Design review of the part built by this model. Coordinates are the model's own, in mm. A direction names the side the tool comes from. Give positions to 0.01 mm unless a question says otherwise; leave off trailing zeros. Order: outer loops, then holes, each group sorted by start corner. A loop starts at its lowest first (then second) coordinate and runs counter-clockwise, first axis right, second up. Notation, with made-up numbers: M 46,44 L 70,44 A13 cw 70,48 Z; hole C 7.5,46.5 d6. An arc over 180 degrees is marked long. Answer as a JSON object with one key per item and string values.
from build123d import *

# Parameters (mm, degrees)
BOX_W           = 67
BOX_H           = 24.4
BOX_DEPTH       = 10.5
THICKNESS_T     = 1.2
SKETCH_W        = 8
SKETCH_H        = 4.3
POCKET_DEPTH    = 5
SKETCH001_W     = 15.5
SKETCH001_H     = 3.2
POCKET001_DEPTH = 5
SKETCH002_W     = 5
SKETCH002_H     = 1
PAD_DEPTH       = 0.5
SKETCH003_W     = 5
SKETCH003_H     = 1
PAD001_DEPTH    = 0.5
CHAMFER_SIZE    = 0.4
CHAMFER001_SIZE = 0.4
CHAMFER002_SIZE = 0.4
CHAMFER003_SIZE = 0.4


with BuildPart() as part:
    # Box → Box (new body)
    with BuildSketch(Plane.XY):
        with Locations((33.5, 12.2)):
            Rectangle(BOX_W, BOX_H)
    extrude(amount=BOX_DEPTH)

    # Thickness
    thickness_openings = [part.faces().sort_by_distance(p)[0] for p in [
        (33.5, 12.2, 10.5),
    ]]
    offset(amount=THICKNESS_T, openings=thickness_openings)

    # Sketch (on Face14 of Thickness) → Pocket (cut)
    with BuildSketch(Plane.XZ.offset(1.2)):
        with Locations((21.188957, 4.340102)):
            Rectangle(SKETCH_W, SKETCH_H)
    extrude(amount=-POCKET_DEPTH, mode=Mode.SUBTRACT)

    # Sketch001 (on Face17 of Pocket) → Pocket001 (cut)
    with BuildSketch(Plane.YZ.offset(68.2)):
        with Locations((15.481014, 3.816542)):
            Rectangle(SKETCH001_W, SKETCH001_H)
    extrude(amount=-POCKET001_DEPTH, mode=Mode.SUBTRACT)

    # Sketch002 (on Face2 of Pocket001) → Pad (join)
    with BuildSketch(Plane.XZ):
        with Locations((7.5565, 3.152776)):
            Rectangle(SKETCH002_W, SKETCH002_H)
        with Locations((62.523926, 3.21387)):
            Rectangle(SKETCH002_W, SKETCH002_H)
    extrude(amount=-PAD_DEPTH)

    # Sketch003 (on Face5 of Pad) → Pad001 (join)
    with BuildSketch(Plane(origin=(0, 24.4, 0), x_dir=(-1, 0, 0), z_dir=(0, 1, 0))):
        with Locations((-57.564125, 3.224103)):
            Rectangle(SKETCH003_W, SKETCH003_H)
        with Locations((-12.49075, 3.224103)):
            Rectangle(SKETCH003_W, SKETCH003_H)
    extrude(amount=-PAD001_DEPTH)

    # Chamfer
    chamfer_edges = [part.edges().sort_by_distance(p)[0] for p in [
        (12.49075, 23.9, 3.724103),
    ]]
    chamfer(chamfer_edges, length=CHAMFER_SIZE)

    # Chamfer001
    chamfer001_edges = [part.edges().sort_by_distance(p)[0] for p in [
        (57.564125, 23.9, 3.724103),
    ]]
    chamfer(chamfer001_edges, length=CHAMFER001_SIZE)

    # Chamfer002
    chamfer002_edges = [part.edges().sort_by_distance(p)[0] for p in [
        (62.523926, 0.5, 3.71387),
    ]]
    chamfer(chamfer002_edges, length=CHAMFER002_SIZE)

    # Chamfer003
    chamfer003_edges = [part.edges().sort_by_distance(p)[0] for p in [
        (7.5565, 0.5, 3.652776),
    ]]
    chamfer(chamfer003_edges, length=CHAMFER003_SIZE)


solid = part.part
(1) We need section A-A (z = 7.75). Write out the cut boundary in (x, y), plus the area to 3 significant figures.
Checked values:
{"outline": "M -1.2,0 A1.2 ccw 0,-1.2 L 67,-1.2 A1.2 ccw 68.2,0 L 68.2,24.4 A1.2 ccw 67,25.6 L 0,25.6 A1.2 ccw -1.2,24.4 Z; hole M 0,0 L 67,0 L 67,24.4 L 0,24.4 Z", "area": "224 mm^2"}
(2) Insertion check: pin 1 (1.3 mm diameter, centred on y = -0.5, z = 5, fed in from +X). The pin has a flat end and moves straight along its axis. Give the tip position at first contact, or say it passes through.
Checked values:
{"pin 1": "stops at x = 68.2"}
(3) Tool access review of faces 4 (the flat face through (25.189, -1, 4)), 5 (the flat face through (23, 25, 10.5)), 6 (the flat face through (68, 15, 5.417)), 7 (the flat face through (0, 12, 5)): name each direction out of +Z, -Z, +X, -X, +Y, -Y from which nothing blocks a thin tool from reaching the whole face with its end or side.
Checked values:
{"face 4": "-Y", "face 5": "+Z, +X, -X, +Y, -Y", "face 6": "+X", "face 7": "+Z"}
(4) Draft analysis for pull direction Z (two halves, no side actions). For faces 1 (the flat face through (67, 12, 6)), 2 (the cylindrical face through (33.969, -0.858, -0.839)), 3 (the flat face through (21, -1, 6.49)), state which applies: +Z half, -Z half, draft (parallel to the pull), parting line (faces both ways), or undercut.
Checked values:
{"face 1": "draft", "face 2": "-Z half", "face 3": "undercut"}
(5) We need section D-D (y = 4.75). Write out the cut boundary in (x, z).
Checked values:
{"outline": "M -1.2,0 A1.2 ccw 0,-1.2 L 67,-1.2 A1.2 ccw 68.2,0 L 68.2,10.5 L 67,10.5 L 67,0 L 0,0 L 0,10.5 L -1.2,10.5 Z"}
(6) We need section B-B (y = 16.75). Write out the cut boundary in (x, z).
Checked values:
{"outline": "M -1.2,0 A1.2 ccw 0,-1.2 L 67,-1.2 A1.2 ccw 68.2,0 L 68.2,2.22 L 67,2.22 L 67,0 L 0,0 L 0,10.5 L -1.2,10.5 Z; M 67,5.42 L 68.2,5.42 L 68.2,10.5 L 67,10.5 Z"}
(7) To check wall thickness, follow L1, parallel to X at y = 3.25, z = 7.5; L2, parallel to Y at x = 33.5, z = 7.75; L3, parallel to X at y = 14, z = 3.25. State the ranges of each line that lie inside material, in increasing order. Write a range as from..to.
Checked values:
{"L1": "x = -1.2..0, 67..68.2", "L2": "y = -1.2..0, 24.4..25.6", "L3": "x = -1.2..0"}
(8) We need section C-C (x = 18.5). Write out the cut boundary in (y, z).
Checked values:
{"outline": "M -1.2,0 A1.2 ccw 0,-1.2 L 24.4,-1.2 A1.2 ccw 25.6,0 L 25.6,10.5 L 24.4,10.5 L 24.4,0 L 0,0 L 0,2.19 L -1.2,2.19 Z; M -1.2,6.49 L 0,6.49 L 0,10.5 L -1.2,10.5 Z"}
